Design review of the part built by this model. Coordinates are the model's own, in mm. Face numbers are marked on the shaded views. Round coordinates to 2 decimals unless told otherwise and drop trailing zeros.
from build123d import *

# Parameters (mm, degrees)
SKETCH1_R           = 50
BOSS_EXTRUDE1_DEPTH = 30
SKETCH2_R           = 5
CUT_EXTRUDE1_DEPTH  = 31
CUT_EXTRUDE10_DEPTH = 31
CIRPATTERN1_COUNT   = 12
FILLET1_R           = 10


with BuildPart() as part:
    # Sketch1 → Boss-Extrude1 (new body)
    with BuildSketch(Plane(origin=(0, 0, 0), x_dir=(0, 0, -1), z_dir=(1, 0, 0))):
        Circle(SKETCH1_R)
    extrude(amount=BOSS_EXTRUDE1_DEPTH)

    # Sketch2 → Cut-Extrude1 (cut, through all)
    with BuildSketch(Plane(origin=(30, 0, 0), x_dir=(0, 0, -1), z_dir=(1, 0, 0))):
        Circle(SKETCH2_R)
    extrude(amount=-CUT_EXTRUDE1_DEPTH, mode=Mode.SUBTRACT)

    # Sketch3 → Cut-Extrude10 (cut, through all)
    with BuildSketch(Plane(origin=(30, 0, 0), x_dir=(0, 0, -1), z_dir=(1, 0, 0))):
        with BuildLine():
            Line((0, -30), (0, -10))
            ThreePointArc((0, -10), (-0.526234368, -9.98614427), (-1.051010465, -9.944615478))
            Line((-1.051010465, -9.944615478), (-5.216763219, -29.542941315))
            ThreePointArc((-5.216763219, -29.542941315), (-2.618373595, -29.885516889), (0, -30))
        make_face()
    cut_extrude10 = extrude(amount=-CUT_EXTRUDE10_DEPTH, mode=Mode.SUBTRACT)

    # CirPattern1: Cut-Extrude10 ×12 about axis
    cirpattern1_axis = Axis((0, 0, 0), (1, 0, 0))
    for i in range(1, CIRPATTERN1_COUNT):
        add(cut_extrude10.rotate(cirpattern1_axis, i * 360 / CIRPATTERN1_COUNT), mode=Mode.SUBTRACT)

    # Fillet1
    fillet1_edges = [part.edges().sort_by_distance(p)[0] for p in [
        (0, 0, 50),
        (30, 0, 50),
    ]]
    fillet(fillet1_edges, radius=FILLET1_R)


solid = part.part
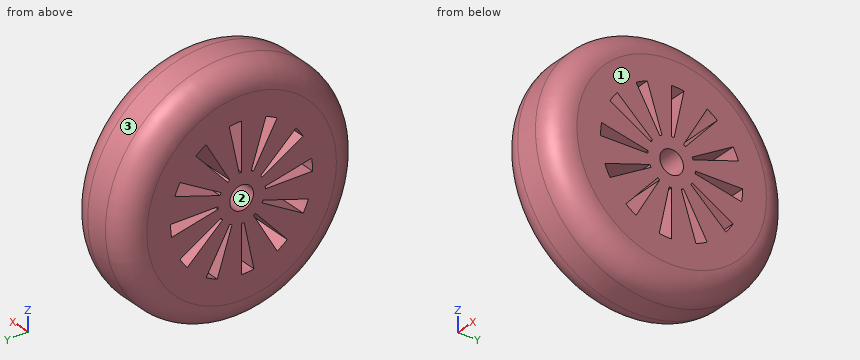
1) The part is to be moulded in two halves that separate along Y. For the marked faces 1, 2 and 3, say which applies: released by +Y, released by -Y, zero draft, split by the parting line, or undercut.
Results:
face 1: zero draft
face 2: undercut
face 3: split by the parting line
2) To check wall thickness, follow line 1 along Y through (x, z) = (9, -19); line 2 along Z through (x, y) = (8.5, -11); line 3 along Z through (x, y) = (15.5, -21). State the ranges of each line that lie inside material, in increasing order.
Results:
line 1: y = -46.2 to -15.71, -10.97 to -2.98, 0 to 7.27, 10.97 to 22.66, 23.22 to 46.2
line 2: z = -48.66 to -19.05, -13.77 to -6.35, -4.67 to 0, 1.28 to 6.35, 8.51 to 19.05, 27.91 to 48.66
line 3: z = -45.38 to -12.12, -7.92 to 0, 3.4 to 12.12, 17.51 to 45.38
3) Take a section at A-A on x = 17.5. State how many separate pieces and enclosed holes the cut face has, plus the area to 3 significant figures.
Results:
separate pieces: 1
enclosed holes: 13
area: 7,020 mm2
4) Clearance check with flat-ended pins moving along their axes: P1, Ø16, axis at x = 19.5, y = 16.5, coming from the -Z side; P2, Ø4, axis at x = 21, y = -25.5, coming from the -Z side; P3, Ø1.5, axis at x = 10, y = 22, coming from the +Z side. State where each tip first meets the part, or that it passes through.
Results:
P1: stops at z = -49.27
P2: stops at z = -44.09
P3: stops at z = 45.26
